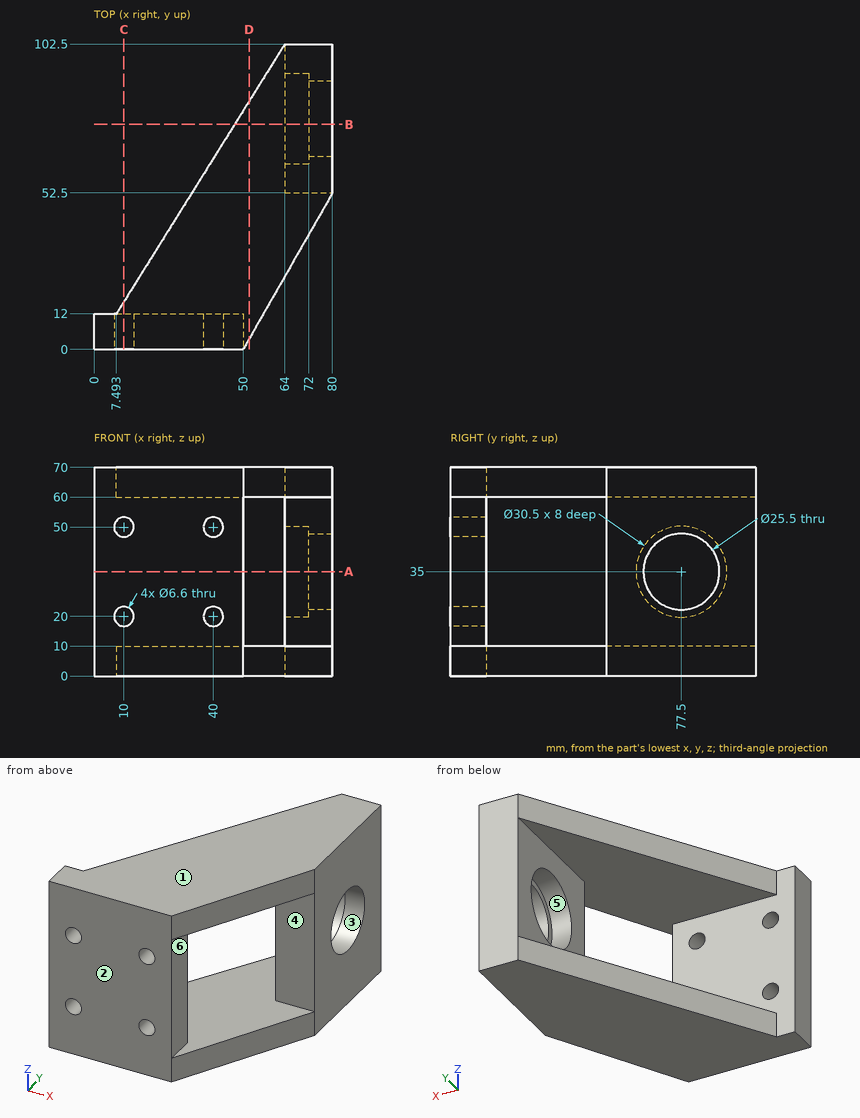
Study the drawing (mm; zero at the part's minimum x, y, z) and answer. A direction names the side the tool comes from. Give positions to 0.01 mm unless a question says otherwise; leave off trailing zeros. Write each loop counter-clockwise with the first axis right and the second up, starting at its lowest first coordinate (ties: lowest second). Pieces come first, ordered by that corner, then holes.
Item 1: Which of the six approach directions +Z, -Z, +X, -X, +Y, -Y give full straight-line access (tool end or side, diameter ignored) to the marked faces 4, 5 and 6?
Item 2: Find the intervals of material crossed by line 1 along X through (y, z) = (3.25, 20); line 2 along Z through (x, y) = (51.5, 5.5); line 3 along Z through (x, y) = (76, 77), in increasing order.
Item 3: Section D-D, the plane x = 52 is taken. Write down the section's boundary in (y, z).
Item 4: Section B-B, the plane y = 75.5 is taken. Write down the section's boundary in (x, z), plus the area to 3 significant figures.
Item 5: Section A-A, the plane z = 35 is taken. Write down the section's boundary in (x, y), plus the area to 3 significant figures.
Item 6: Determine the mould class of the marked faces 1, 2 and 3 for opening direction Z: released by +Z, released by -Z, zero draft, split by the parting line, or undercut.
Item 7: Section C-C, the plane x = 10 is taken. Write down the section's boundary in (y, z) (1 decimal), plus the area to 3 significant figures.
Item 8: Flat-ended cylindrical pins translate along their axes: P1, Ø4, axis at x = 10, z = 50, coming from the -Y side; P2, Ø17.5, axis at x = 72.5, z = 30, coming from the -Y side; P3, Ø9.5, axis at y = 5.5, z = 34, coming from the +X side; P4, Ø6, axis at x = 49, z = 8, coming from the +Y side. Find the tip coordinate at first contact, or state that the pin passes through.
Completed:
1. face 4: +X, -X, -Y
1. face 5: -X
1. face 6: +X, +Y, -Y
2. line 1: x = 0 to 6.7, 13.3 to 36.7, 43.3 to 50
2. line 2: z = 0 to 10, 60 to 70
2. line 3: z = 0 to 22.26, 47.74 to 70
3. outline: (3.5, 0) - (83.28, 0) - (83.28, 10) - (3.5, 10) - close; (3.5, 60) - (83.28, 60) - (83.28, 70) - (3.5, 70) - close
4. outline: (47.14, 0) - (80, 0) - (80, 22.41) - (72, 22.41) - (72, 19.88) - (64, 19.88) - (64, 10) - (47.14, 10) - close; (47.14, 60) - (64, 60) - (64, 50.12) - (72, 50.12) - (72, 47.59) - (80, 47.59) - (80, 70) - (47.14, 70) - close
4. area: 1,010 mm2
5. outline: (0, 0) - (50, 0) - (50, 12) - (0, 12) - close; (64, 52.5) - (80, 52.5) - (80, 64.75) - (72, 64.75) - (72, 62.25) - (64, 62.25) - close; (64, 92.75) - (72, 92.75) - (72, 90.25) - (80, 90.25) - (80, 102.5) - (64, 102.5) - close
5. area: 952 mm2
6. face 1: released by +Z
6. face 2: zero draft
6. face 3: undercut
7. outline: (0, 0) - (16, 0) - (16, 10) - (12, 10) - (12, 16.7) - (0, 16.7) - close; (0, 23.3) - (12, 23.3) - (12, 46.7) - (0, 46.7) - close; (0, 53.3) - (12, 53.3) - (12, 60) - (16, 60) - (16, 70) - (0, 70) - close
7. area: 762 mm2
8. P1: passes through
8. P2: stops at y = 52.5
8. P3: stops at x = 50
8. P4: stops at y = 83.28
